```python
from build123d import *

# Parameters (mm, degrees)
SKETCH7_W           = 40
SKETCH7_H           = 40
BOSS_EXTRUDE1_DEPTH = 14
LOFT1_START         = -20
LOFT1_DEPTH         = 40
SKETCH16_W          = 49.026286786
SKETCH16_H          = 65.242270374
SKETCH16_R          = 20
CUT_EXTRUDE3_DEPTH  = 6
SKETCH17_W          = 40
SKETCH17_H          = 8
BOSS_EXTRUDE5_DEPTH = 18
SKETCH10_R          = 2.25
CUT_EXTRUDE1_DEPTH  = 25
CHAMFER1_SIZE       = 2.5
FILLET3_R           = 20
SKETCH11_W          = 46.2
SKETCH11_H          = 14
BOSS_EXTRUDE6_DEPTH = 43
FILLET9_R           = 2.5
SKETCH20_W          = 40.6
SKETCH20_H          = 4.4
CUT_EXTRUDE4_DEPTH  = 40
SKETCH22_R          = 1.7
CUT_EXTRUDE5_DEPTH  = 30
FILLET11_R          = 2
CUT_EXTRUDE6_DEPTH  = 4
SKETCH24_R          = 3
CUT_EXTRUDE7_DEPTH  = 3


# Read off the part's stored shape, not the designer's step: Loft1
with BuildPart() as part:
    # Sketch7 → Boss-Extrude1 (new body)
    with BuildSketch(Plane.XY):
        Rectangle(SKETCH7_W, SKETCH7_H)
    extrude(amount=BOSS_EXTRUDE1_DEPTH)

    # Loft1 outline → Loft1 (add)
    with BuildSketch(Plane.YZ.offset(LOFT1_START)):
        with BuildLine():
            add(Edge.make_bspline(
                [(-38, 18), (-31.853637028, 18), (-26.146362972, 14), (-20, 14)],
                knots=[0, 0, 0, 0, 1, 1, 1, 1], degree=3))
            Line((-38, 18), (-38, 10))
            add(Edge.make_bspline(
                [(-38, 10), (-31.853637028, 10), (-26.146362972, 6), (-20, 6)],
                knots=[0, 0, 0, 0, 1, 1, 1, 1], degree=3))
            Line((-20, 6), (-20, 14))
        make_face()
    extrude(amount=LOFT1_DEPTH)

    # Sketch16 → Cut-Extrude3 (cut)
    with BuildSketch(Plane(origin=(0, 0, 0), x_dir=(-1, 0, 0), z_dir=(0, 0, -1))):
        Rectangle(SKETCH16_W, SKETCH16_H)
        Circle(SKETCH16_R, mode=Mode.SUBTRACT)
    extrude(amount=-CUT_EXTRUDE3_DEPTH, mode=Mode.SUBTRACT)

    # Sketch17 → Boss-Extrude5 (add)
    with BuildSketch(Plane(origin=(0, -38, 0), x_dir=(-1, 0, 0), z_dir=(0, -1, 0))):
        with Locations((0, -14)):
            Rectangle(SKETCH17_W, SKETCH17_H)
    extrude(amount=BOSS_EXTRUDE5_DEPTH)

    # Sketch10 → Cut-Extrude1 (cut)
    with BuildSketch(Plane.XY.offset(14)):
        with Locations((-7.00009521, 12.124420806)):
            Circle(SKETCH10_R)
        with Locations((6.99990479, 12.124420806)):
            Circle(SKETCH10_R)
        with Locations((13.99990479, 6.5153e-05)):
            Circle(SKETCH10_R)
        with Locations((6.99990479, -12.1242905)):
            Circle(SKETCH10_R)
        with Locations((-7.00009521, -12.1242905)):
            Circle(SKETCH10_R)
        with Locations((-14.00009521, 6.5153e-05)):
            Circle(SKETCH10_R)
    extrude(amount=-CUT_EXTRUDE1_DEPTH, mode=Mode.SUBTRACT)

    # Chamfer1
    chamfer1_edges = [part.edges().sort_by_distance(p)[0] for p in [
        (4.74990479, 12.124420806, 14),
        (-9.25009521, 12.124420806, 14),
        (-16.25009521, 6.5153e-05, 14),
        (-9.25009521, -12.1242905, 14),
        (4.74990479, -12.1242905, 14),
        (11.74990479, 6.5153e-05, 14),
    ]]
    chamfer(chamfer1_edges, length=CHAMFER1_SIZE)

    # Fillet3
    fillet3_edges = [part.edges().sort_by_distance(p)[0] for p in [
        (20, 20, 10),
        (-20, 20, 10),
    ]]
    fillet(fillet3_edges, radius=FILLET3_R - 0.0001)  # a hair under: the kernel refuses the full size

    # Sketch11 → Boss-Extrude6 (add)
    with BuildSketch(Plane(origin=(0, -56, -3.472963553), x_dir=(1, 0, 0), z_dir=(0, 1, 0))):
        with Locations((0, -14.472963553)):
            Rectangle(SKETCH11_W, SKETCH11_H)
    extrude(amount=-BOSS_EXTRUDE6_DEPTH)

    # Fillet9
    fillet9_edges = [part.edges().sort_by_distance(p)[0] for p in [
        (0, -56, 10),
        (-20, -56, 14),
        (20, -56, 14),
    ]]
    fillet(fillet9_edges, radius=FILLET9_R)

    # Sketch20 → Cut-Extrude4 (cut)
    with BuildSketch(Plane.XZ.offset(99)):
        with Locations((0, 11)):
            Rectangle(SKETCH20_W, SKETCH20_H)
    extrude(amount=-CUT_EXTRUDE4_DEPTH, mode=Mode.SUBTRACT)

    # Sketch22 → Cut-Extrude5 (cut)
    with BuildSketch(Plane.XY):
        with Locations(Location((11, -68.5, 0), (0, 0, 180))):
            Circle(SKETCH22_R)
        with Locations(Location((11, -90.5, 0), (0, 0, 180))):
            Circle(SKETCH22_R)
        with Locations(Location((-11, -90.5, 0), (0, 0, 180))):
            Circle(SKETCH22_R)
        with Locations(Location((-11, -68.5, 0), (0, 0, 180))):
            Circle(SKETCH22_R)
    extrude(amount=CUT_EXTRUDE5_DEPTH, mode=Mode.SUBTRACT)

    # Fillet11
    fillet11_edges = [part.edges().sort_by_distance(p)[0] for p in [
        (-23.1, -77.5, 18),
        (-23.1, -77.5, 4),
        (23.1, -77.5, 18),
        (23.1, -77.5, 4),
    ]]
    fillet(fillet11_edges, radius=FILLET11_R)

    # Sketch23 → Cut-Extrude6 (cut)
    with BuildSketch(Plane.XY.offset(18)):
        Polygon((-11, -65.324573519), (-13.75, -66.91228676), (-13.75, -70.08771324), (-11, -71.675426481), (-8.25, -70.08771324), (-8.25, -66.91228676), align=None)
        Polygon((11, -65.324573519), (8.25, -66.91228676), (8.25, -70.08771324), (11, -71.675426481), (13.75, -70.08771324), (13.75, -66.91228676), align=None)
        Polygon((11, -87.324573519), (8.25, -88.91228676), (8.25, -92.08771324), (11, -93.675426481), (13.75, -92.08771324), (13.75, -88.91228676), align=None)
        Polygon((-11, -87.324573519), (-13.75, -88.91228676), (-13.75, -92.08771324), (-11, -93.675426481), (-8.25, -92.08771324), (-8.25, -88.91228676), align=None)
    extrude(amount=-CUT_EXTRUDE6_DEPTH, mode=Mode.SUBTRACT)

    # Sketch24 → Cut-Extrude7 (cut)
    with BuildSketch(Plane(origin=(0, 0, 4), x_dir=(-1, 0, 0), z_dir=(0, 0, -1))):
        with Locations((-11, -68.5)):
            Circle(SKETCH24_R)
        with Locations((11, -68.5)):
            Circle(SKETCH24_R)
        with Locations((11, -90.5)):
            Circle(SKETCH24_R)
        with Locations((-11, -90.5)):
            Circle(SKETCH24_R)
    extrude(amount=-CUT_EXTRUDE7_DEPTH, mode=Mode.SUBTRACT)


solid = part.part
```
The model under review builds one solid part; all positions refer to its coordinate system, in mm. A direction names the side the tool comes from. Give positions to 0.01 mm unless a question says otherwise; leave off trailing zeros. Write each loop counter-clockwise with the first axis right and the second up, starting at its lowest first coordinate (ties: lowest second). Pieces come first, ordered by that corner, then holes. Notation, with made-up numbers: (72, 6) - (96, 6) arc R15 ccw to (96, 11) - close; hole circle Ø6 at (82, 57.5). An arc over 180 degrees is marked (long way). Answer in a Markdown table with one row per item. Add a question column.
1. Insertion check: P1, Ø8, axis at x = 14, z = 15, coming from the +Y side; P2, Ø5, axis at x = 11, y = -90.5, coming from the -Z side; P3, Ø5, axis at x = -11, y = -90.5, coming from the +Z side; P4, Ø2, axis at x = 13.5, z = 9, coming from the -Y side. Each pin has a flat end and moves straight along its axis. Give the tip position at first contact, or say it passes through.
2. We need section B-B on z = 1.5. Write out the cut boundary in (x, y), then the cut area to 3 significant figures.
3. Wall thickness on line 1 along X through (y, z) = (-68.5, 13.8); line 2 along Z through (x, y) = (20, -88.5); line 3 along X through (y, z) = (11, 13.25): over which ranges is each line inside the solid? List them lowest first. Write a range as [from, to].
4. Draft analysis for pull direction Z (two halves, no side actions). For faces 1 (the flat face through (0, -59, 11)), 2 (the flat face through (-13, -68, 7)), 3 (the flat face through (0, -4, 14)), 4 (the flat face through (-9.606, -88.13, 16.028)), state which applies: +Z half, -Z half, draft (parallel to the pull), parting line (faces both ways), or undercut.
5. We need section A-A on y = -90.5. State how many separate pieces and enclosed holes the cut face has, then the cut area to 3 significant figures.
6. Tool access review of faces 5 (the flat face through (0, -79, 8.8)), 6 (the flat face through (9.606, -92.87, 16.028)), 7 (the cylindrical face through (11.65, -71.43, 5.48)): name each direction out of +Z, -Z, +X, -X, +Y, -Y from which nothing blocks a thin tool from reaching the whole face with its end or side.
Ans:
| question | item | result |
|---|---|---|
| 1 | P1 | stops at y = 17.25 |
| 1 | P2 | stops at z = 7 |
| 1 | P3 | stops at z = 14 |
| 1 | P4 | stops at y = -99 |
| 2 | outline | circle Ø40 at (0, 0); hole circle Ø4.5 at (-14, 0); hole circle Ø4.5 at (-7, -12.12); hole circle Ø4.5 at (-7, 12.12); hole circle Ø4.5 at (7, -12.12); hole circle Ø4.5 at (7, 12.12); hole circle Ø4.5 at (14, 0) |
| 2 | area | 1,160 mm^2 |
| 3 | line 1 | x = [-23.1, -12.7], [-9.3, 9.3], [12.7, 23.1] |
| 3 | line 2 | z = [4, 8.8], [13.2, 18] |
| 3 | line 3 | x = [-16.7, -10.84], [-3.16, 3.16], [10.84, 16.7] |
| 4 | face 1 | undercut |
| 4 | face 2 | -Z half |
| 4 | face 3 | +Z half |
| 4 | face 4 | draft |
| 5 | separate pieces | 4 |
| 5 | enclosed holes | 0 |
| 5 | area | 367 mm^2 |
| 6 | face 5 | -Y |
| 6 | face 6 | +Z |
| 6 | face 7 | -Z |
